Can you work these out from the model? Positions are in its coordinate system, mm. A direction names the side the tool comes from. Give positions to 0.01 mm unless a question says otherwise; leave off trailing zeros. Order: outer loops, then holes, each group sorted by start corner. A loop starts at its lowest first (then second) coordinate and runs counter-clockwise, first axis right, second up. Notation, with made-up numbers: (-16, 54) -> (12, 54) arc R27 cw to (12, 93) -> close; hole circle Ø4 at (83, -1). An arc over 180 degrees is marked (long way). Answer as a JSON object with one key per item and string values.
Autodesk Inventor part; units mm, degrees
ref_plane "YZ Plane" through (0, 0, 0) normal (1, 0, 0) x (0, 1, 0)
ref_plane "XZ Plane" through (0, 0, 0) normal (0, 1, 0) x (-1, 0, 0)
ref_plane "XY Plane" through (0, 0, 0) normal (0, 0, 1) x (1, 0, 0)
sketch "Sketch1" plane through (0, 0, 0) normal (0, 1, 0) x (-1, 0, 0)
  arc A0 (-2.4004, 17.3346) -> (-2.3887, -17.3362) centre (0, 0) ccw
  arc A1 (-6.5816, 21.5159) -> (-6.5714, -21.519) centre (0, 0) ccw
  circle A2 centre (0, 10) radius 1
  circle A3 centre (0, -10) radius 1
  arc A4 (-2.3933, 7.4462) -> (2.2712, 12.663) centre (0, 10) ccw
  arc A5 (2.4002, -12.5474) -> (-2.4749, -7.5251) centre (0, -10) ccw
  line L0 (-8, 55) -> (-16, 55)
  line L1 (-16, -55) -> (-8, -55)
  line L2 (-8, -55) -> (-8, -22.9476)
  line L3 (-8, 22.9342) -> (-8, 55)
  line L4 (-16, -23.152) -> (-16, -55)
  line L5 (-8, 22.9342) -> (2.5474, 12.3868)
  line L6 (-8, 22.9342) -> (6.9163, 22.9342) construction
  line L7 (2.5474, -12.4002) -> (-8, -22.9476)
  line L8 (-2.4749, -7.5251) -> (-9.5993, -14.6496)
  circle A6 centre (-12, -50.8) radius 1.5
  circle A7 centre (-12, -38.1) radius 1.5
  circle A8 centre (-12, 50.8) radius 1.5
  circle A9 centre (-12, 38.1) radius 1.5
  line L9 (-16, 55) -> (-16, 21.0529)
  line L10 (-9.5993, -14.6496) -> (-16, -21.0503)
  line L11 (-16, -21.0503) -> (-16, -23.152)
  line L12 (-2.3933, 7.4462) -> (-16, 21.0529)
  line L13 (0, 14.9342) -> (-4.9407, 9.9935)
  line L14 (0, -14.9476) -> (-4.9487, -9.9989)
  point P0 (-9.5889, -14.6391)
  point P1 (-9.5873, 14.6401)
  dimension "d7" = 35
  dimension "d8" = 45
  dimension "d9" = 2
  dimension "d10" = 2
  dimension "d11" = 10
  dimension "d12" = 10
  dimension "d13" = 7
  dimension "d14" = 7
  dimension "d19" = 8
  dimension "d20" = 110
  dimension "d21" = 8
  dimension "d22" = 55
  dimension "d23" = 45
  dimension "d25" = 3
  dimension "d26" = 3
  dimension "d27" = 3
  dimension "d28" = 3
  dimension "d29" = 38.1
  dimension "d31" = 50.8
sketch "Sketch2" plane through (0, 0, 0) normal (0, 1, 0) x (-1, 0, 0)
  arc A0 (-2.4004, 17.3346) -> (-2.3887, -17.3362) centre (0, 0) ccw
  arc A1 (-6.5816, 21.5159) -> (-6.5714, -21.519) centre (0, 0) ccw
  circle A2 centre (0, 10) radius 1.13
  circle A3 centre (0, -10) radius 1.13
  arc A4 (-2.3933, 7.4462) -> (2.2712, 12.663) centre (0, 10) ccw
  arc A5 (2.4002, -12.5474) -> (-2.4749, -7.5251) centre (0, -10) ccw
  line L0 (-8, 55) -> (-16, 55)
  line L1 (-16, -55) -> (-8, -55)
  line L2 (-8, -55) -> (-8, -22.9476)
  line L3 (-8, 22.9342) -> (-8, 55)
  line L4 (-16, -23.152) -> (-16, -55)
  line L5 (-8, 22.9342) -> (2.5474, 12.3868)
  line L6 (-8, 22.9342) -> (6.9163, 22.9342) construction
  line L7 (2.5474, -12.4002) -> (-8, -22.9476)
  line L8 (-2.4749, -7.5251) -> (-9.5993, -14.6496)
  circle A6 centre (-12, -50.8) radius 1.5
  circle A7 centre (-12, -38.1) radius 1.5
  circle A8 centre (-12, 50.8) radius 1.5
  circle A9 centre (-12, 38.1) radius 1.5
  line L9 (-16, 55) -> (-16, 21.0529)
  line L10 (-9.5993, -14.6496) -> (-16, -21.0503)
  line L11 (-16, -21.0503) -> (-16, -23.152)
  line L12 (-2.3933, 7.4462) -> (-16, 21.0529)
  line L13 (0, 14.9342) -> (-4.9407, 9.9935)
  line L14 (0, -14.9476) -> (-4.9487, -9.9989)
  dimension "d54" = 35
  dimension "d55" = 45
  dimension "d56" = 2.26
  dimension "d57" = 2.26
  dimension "d58" = 10
  dimension "d59" = 10
  dimension "d60" = 7
  dimension "d61" = 7
  dimension "d62" = 8
  dimension "d63" = 110
  dimension "d64" = 8
  dimension "d65" = 55
  dimension "d66" = 45
  dimension "d67" = 3
  dimension "d68" = 3
  dimension "d69" = 3
  dimension "d70" = 3
  dimension "d71" = 38.1
  dimension "d72" = 50.8
sketch "Sketch3" plane through (0, 0, 0) normal (0, 1, 0) x (-1, 0, 0)
  arc A0 (-2.4004, 17.3346) -> (-2.3887, -17.3362) centre (0, 0) ccw
  arc A1 (-6.5816, 21.5159) -> (-6.5714, -21.519) centre (0, 0) ccw
  circle A2 centre (0, 10) radius 1
  circle A3 centre (0, -10) radius 1
  arc A4 (-2.3933, 7.4462) -> (2.2712, 12.663) centre (0, 10) ccw
  arc A5 (2.4002, -12.5474) -> (-2.4749, -7.5251) centre (0, -10) ccw
  line L0 (-8, 55) -> (-16, 55)
  line L1 (-16, -55) -> (-8, -55)
  line L2 (-8, -55) -> (-8, -22.9476)
  line L3 (-8, 22.9342) -> (-8, 55)
  line L4 (-16, -23.152) -> (-16, -55)
  line L5 (-8, 22.9342) -> (2.5474, 12.3868)
  line L6 (-8, 22.9342) -> (6.9163, 22.9342) construction
  line L7 (2.5474, -12.4002) -> (-8, -22.9476)
  line L8 (-2.4749, -7.5251) -> (-9.5993, -14.6496)
  circle A6 centre (-12, -50.8) radius 1.5
  circle A7 centre (-12, -38.1) radius 1.5
  circle A8 centre (-12, 50.8) radius 1.5
  circle A9 centre (-12, 38.1) radius 1.5
  line L9 (-16, 55) -> (-16, 21.0529)
  line L10 (-9.5993, -14.6496) -> (-16, -21.0503)
  line L11 (-16, -21.0503) -> (-16, -23.152)
  line L12 (-2.3933, 7.4462) -> (-16, 21.0529)
  line L13 (0, 14.9342) -> (-4.9407, 9.9935)
  line L14 (0, -14.9476) -> (-4.9487, -9.9989)
  point P0 (-9.5889, -14.6391)
  point P1 (-9.5873, 14.6401)
  point P2 (-13.1831, -18.2334)
  point P3 (-13.1816, 18.2345)
  dimension "d92" = 35
  dimension "d93" = 45
  dimension "d94" = 2
  dimension "d95" = 2
  dimension "d96" = 10
  dimension "d97" = 10
  dimension "d98" = 7
  dimension "d99" = 7
  dimension "d100" = 8
  dimension "d101" = 110
  dimension "d102" = 8
  dimension "d103" = 55
  dimension "d104" = 45
  dimension "d105" = 3
  dimension "d106" = 3
  dimension "d107" = 3
  dimension "d108" = 3
  dimension "d109" = 38.1
  dimension "d110" = 50.8
sketch "Sketch4" plane through (0, 0, 0) normal (0, 1, 0) x (-1, 0, 0)
  arc A0 (-2.4004, 17.3346) -> (-2.3887, -17.3362) centre (0, 0) ccw
  arc A1 (-6.5816, 21.5159) -> (-6.5714, -21.519) centre (0, 0) ccw
  circle A2 centre (0, 10) radius 1
  circle A3 centre (0, -10) radius 1
  arc A4 (-2.3933, 7.4462) -> (2.2712, 12.663) centre (0, 10) ccw
  arc A5 (2.4002, -12.5474) -> (-2.4749, -7.5251) centre (0, -10) ccw
  line L0 (-8, 55) -> (-16, 55)
  line L1 (-16, -55) -> (-8, -55)
  line L2 (-8, -55) -> (-8, -22.9476)
  line L3 (-8, 22.9342) -> (-8, 55)
  line L4 (-16, -23.152) -> (-16, -55)
  line L5 (-8, 22.9342) -> (2.5474, 12.3868)
  line L6 (-8, 22.9342) -> (6.9163, 22.9342) construction
  line L7 (2.5474, -12.4002) -> (-8, -22.9476)
  line L8 (-2.4749, -7.5251) -> (-9.5993, -14.6496)
  circle A6 centre (-12, -50.8) radius 1.5
  circle A7 centre (-12, -38.1) radius 1.5
  circle A8 centre (-12, 50.8) radius 1.5
  circle A9 centre (-12, 38.1) radius 1.5
  line L9 (-16, 55) -> (-16, 21.0529)
  line L10 (-9.5993, -14.6496) -> (-16, -21.0503)
  line L11 (-16, -21.0503) -> (-16, -23.152)
  line L12 (-2.3933, 7.4462) -> (-16, 21.0529)
  line L13 (0, 14.9342) -> (-4.9407, 9.9935)
  line L14 (0, -14.9476) -> (-4.9487, -9.9989)
  dimension "d35" = 35
  dimension "d36" = 45
  dimension "d37" = 2
  dimension "d38" = 2
  dimension "d39" = 10
  dimension "d40" = 10
  dimension "d41" = 7
  dimension "d42" = 7
  dimension "d43" = 8
  dimension "d44" = 110
  dimension "d45" = 8
  dimension "d46" = 55
  dimension "d47" = 45
  dimension "d48" = 3
  dimension "d49" = 3
  dimension "d50" = 3
  dimension "d51" = 3
  dimension "d52" = 38.1
  dimension "d53" = 50.8
sketch "Sketch5" plane through (0, 0, 0) normal (0, 1, 0) x (-1, 0, 0)
  arc A0 (-2.4004, 17.3346) -> (-2.3887, -17.3362) centre (0, 0) ccw
  arc A1 (-6.5816, 21.5159) -> (-6.5714, -21.519) centre (0, 0) ccw
  circle A2 centre (0, 10) radius 1
  circle A3 centre (0, -10) radius 1
  arc A4 (-2.3933, 7.4462) -> (2.2712, 12.663) centre (0, 10) ccw
  arc A5 (2.4002, -12.5474) -> (-2.4749, -7.5251) centre (0, -10) ccw
  line L0 (-8, 55) -> (-16, 55)
  line L1 (-16, -55) -> (-8, -55)
  line L2 (-8, -55) -> (-8, -22.9476)
  line L3 (-8, 22.9342) -> (-8, 55)
  line L4 (-16, -23.152) -> (-16, -55)
  line L5 (-8, 22.9342) -> (2.5474, 12.3868)
  line L6 (-8, 22.9342) -> (6.9163, 22.9342) construction
  line L7 (2.5474, -12.4002) -> (-8, -22.9476)
  line L8 (-2.4749, -7.5251) -> (-9.5993, -14.6496)
  circle A6 centre (-12, -50.8) radius 1.5
  circle A7 centre (-12, -38.1) radius 1.5
  circle A8 centre (-12, 50.8) radius 1.5
  circle A9 centre (-12, 38.1) radius 1.5
  line L9 (-16, 55) -> (-16, 21.0529)
  line L10 (-9.5993, -14.6496) -> (-16, -21.0503)
  line L11 (-16, -21.0503) -> (-16, -23.152)
  line L12 (-2.3933, 7.4462) -> (-16, 21.0529)
  line L13 (0, 14.9342) -> (-4.9407, 9.9935)
  line L14 (0, -14.9476) -> (-4.9487, -9.9989)
  point P0 (-9.5873, 14.6401)
  point P1 (-13.1816, 18.2345)
  point P2 (-13.1831, -18.2334)
  point P3 (-9.5889, -14.6391)
  dimension "d73" = 35
  dimension "d74" = 45
  dimension "d75" = 2
  dimension "d76" = 2
  dimension "d77" = 10
  dimension "d78" = 10
  dimension "d79" = 7
  dimension "d80" = 7
  dimension "d81" = 8
  dimension "d82" = 110
  dimension "d83" = 8
  dimension "d84" = 55
  dimension "d85" = 45
  dimension "d86" = 3
  dimension "d87" = 3
  dimension "d88" = 3
  dimension "d89" = 3
  dimension "d90" = 38.1
  dimension "d91" = 50.8
extrude "Extrusion1" add sketch "Sketch2" along normal blind 2 contours L5 A4 L12 L13 | L8 A5 L7 L14
extrude "Extrusion2" add sketch "Sketch1" along normal blind 4 contours L5 L13 L12 A0 | L8 L14 L7 A0
extrude "Extrusion3" add sketch "Sketch3" along normal blind 6 contours A1 L12 L9 L0 L3 L5 | A1 L7 L2 L1 L4 L11 L10
extrude "Extrusion4" add sketch "Sketch4" along normal blind 16 contours A0 L12 A1 L5 | A0 L8 L10 A1 L12 | A0 L7 A1 L10 L8
extrude "Extrusion5" cut sketch "Sketch5" along normal blind 8 contours A0 L8 L10 A1 L12
thread "Thread1"
thread "Thread2"
properties part number "snHeadbarHolder2"
1. If we section it at C-C on y = 14.5: Please give me the cut outline in (x, z).
Worked answers:
{"outline": "(2.39, -17.34) -> (6.57, -21.52) arc R22.5 ccw to (6.58, 21.52) -> (2.4, 17.33) arc R17.5 cw to start"}
2. Will these pins go through, and if not, where does the flat tip stop? pin 1 Ø8 at (y, z) = (5, 38.5) entering from +X; pin 2 Ø4 at (x, z) = (15, 6) entering from -Y; pin 3 Ø2 at (y, z) = (9.5, -1.5) entering from -X; pin 4 Ø1.8 at (x, z) = (12, -38.1) entering from -Y.
Worked answers:
{"pin 1": "x = 16", "pin 2": "y = 8", "pin 3": "x = 17.32", "pin 4": "through"}
3. If we section it at B-B on z = -33.5: Please give me the cut outline in (x, y).
Worked answers:
{"outline": "(8, 0) -> (16, 0) -> (16, 6) -> (8, 6) -> close"}
4. If we section it at A-A on z = -50.8: Please give me the cut outline in (x, y).
Worked answers:
{"outline": "(8, 0) -> (10.5, 0) -> (10.5, 6) -> (8, 6) -> close; (13.5, 0) -> (16, 0) -> (16, 6) -> (13.5, 6) -> close"}
5. If we mould it in two halves opening along X, with no side actions, what happens to faces 1 (the face through (4.078, 6.11, 19.012)), 2 (the face through (-0.61, 0.99, 9.05)), 3 (the face through (12, 3, 55))? For each: +X half, -X half, draft (parallel to the pull), parting line (faces both ways), or undercut.
Worked answers:
{"face 1": "-X half", "face 2": "undercut", "face 3": "draft"}
6. For faces 4 (the face through (11, 0, 31)), 5 (the face through (8, 3, -39)), 6 (the face through (10.613, 3.055, 15.666)), 7 (the face through (-1, 2, -11)), which set-ups out of +Z, -Z, +X, -X, +Y, -Y let a thin tool reach every point of the face, with its end or its side?
Worked answers:
{"face 4": "+Z, -Z, +X, -X, -Y", "face 5": "-Z, -X, +Y, -Y", "face 6": "+X, -Y", "face 7": "-X, +Y"}
7. Please list where these lines run through material, in increasing order: L1, parallel to Z at x = 0, y = 1.4; L2, parallel to Z at x = 11.75, y = 1.5; L3, parallel to Z at x = 12, y = 3.4.
Worked answers:
{"L1": "-14.95 to -11.13, -8.87 to -6.5, 6.5 to 8.87, 11.13 to 14.93", "L2": "-55 to -52.28, -49.32 to -39.58, -36.62 to -16.8, 16.8 to 36.62, 39.58 to 49.32, 52.28 to 55", "L3": "-55 to -52.3, -49.3 to -39.6, -36.6 to -17.05, 17.05 to 36.6, 39.6 to 49.3, 52.3 to 55"}
